Geometry: final body of the model. Coordinates: model frame, mm. A direction names the side the tool comes from. Coordinates: 2 decimals unless noted, no trailing zeros. Write each loop counter-clockwise with the first axis right and the second up, starting at its lowest first coordinate (ties: lowest second). Pieces come first, ordered by that corner, then holes. Notation, with made-up numbers: M 60.5,-12.75 L 108.5,-12.75 A30 ccw 108.5,23.25 Z; hole C 88.25,85.5 d5. An arc over 180 degrees is marked long. Write item = value, one per line. Start each with the question number.
Item 1: Reachability of faces 5 (the flat face through (96.71, 1, 3)), 6 (the flat face through (99, -30.344, 3)), 7 (the flat face through (85, 48.156, 3)) from +Z, -Z, +X, -X, +Y, -Y: full face, straight path, thin tool, end or side. Return the list, or none.
Item 2: First-contact query: pin 1 Ø3 at (x, z) = (85.5, 3.5) entering from -Y; pin 2 Ø1 at (x, z) = (-42.5, 4.5) entering from +Y; pin 3 Ø1.6 at (x, z) = (100, 4) entering from +Y; pin 4 Ø8 at (x, y) = (32.5, 30.5) entering from -Z. Flat tips, straight axial feed; report the tip coordinate or a pass-through.
Item 3: Pull-direction query (X, two-part tool) for faces 1 (the flat face through (-57.29, -20, 3)), 2 (the flat face through (39.21, 25, 3)), 3 (the flat face through (-60, 11.656, 3)), 4 (the flat face through (-31.79, -49, 3)); classes: +X half, -X half, draft (parallel to the pull), parting line (faces both ways), or undercut.
Item 4: Section A-A on y = 26. Output: boundary loops of the cut face in (x, z).
Item 5: Ray query, L1, parallel to Y at x = 43.5, z = 3.95; L2, parallel to X at y = 28, z = 4.05; L3, parallel to Y at x = 53, z = 3.3. Return the intervals inside material, ascending. Write a range as [from, to].
Item 6: Section C-C on z = 1.1. Give the number of separate pieces and of enclosed holes in the cut face, plus the area to 3 significant figures.
Item 7: Section D-D on y = 38.5. Output: boundary loops of the cut face in (x, z), plus the area to 3 significant figures.
Item 8: Section B-B on x = 85. Output: boundary loops of the cut face in (y, z).
from build123d import *

# Parameters (mm, degrees)
CROQUIS2_W              = 21
CROQUIS2_H              = 5.5
CROQUIS2_W_2            = 15.5
SALIENTE_EXTRUIR1_DEPTH = 5.5
CROQUIS3_W              = 21
CROQUIS3_H              = 5.5
CROQUIS3_W_2            = 7.5
SALIENTE_EXTRUIR2_DEPTH = 2.5
CROQUIS4_W              = 5.5
CROQUIS4_H              = 18.5
CROQUIS4_H_2            = 21
SALIENTE_EXTRUIR3_DEPTH = 2.5
CROQUIS5_W              = 10
CROQUIS5_H              = 5.5
CROQUIS5_W_2            = 21
SALIENTE_EXTRUIR4_DEPTH = 2.5
CROQUIS6_W              = 5.5
CROQUIS6_H              = 21
SALIENTE_EXTRUIR5_DEPTH = 2.5


with BuildPart() as part:
    # Croquis2 → Saliente-Extruir1 (new body)
    with BuildSketch(Plane.XY):
        Polygon((-60.290430527, -48.844252157), (-52.790430527, -48.844252157), (-52.790430527, -45.844252157), (-31.790430527, -45.844252157), (-31.790430527, -48.844252157), (-10.790430527, -48.844252157), (-10.790430527, -45.844252157), (10.209569473, -45.844252157), (10.209569473, -48.844252157), (31.209569473, -48.844252157), (31.209569473, -45.844252157), (52.209569473, -45.844252157), (52.209569473, -48.844252157), (73.209569473, -48.844252157), (73.209569473, -45.844252157), (94.209569473, -45.844252157), (96.709569473, -45.844252157), (96.709569473, -30.344252157), (99.709569473, -30.344252157), (99.709569473, -9.344252157), (96.709569473, -9.344252157), (96.709569473, 11.655747843), (99.709569473, 11.655747843), (99.709569473, 32.655747843), (96.709569473, 32.655747843), (96.709569473, 48.155747843), (73.209569473, 48.155747843), (73.209569473, 51.155747843), (52.209569473, 51.155747843), (52.209569473, 48.155747843), (31.209569473, 48.155747843), (31.209569473, 51.155747843), (10.209569473, 51.155747843), (10.209569473, 48.155747843), (-10.790430527, 48.155747843), (-10.790430527, 51.155747843), (-31.790430527, 51.155747843), (-31.790430527, 48.155747843), (-52.790430527, 48.155747843), (-52.790430527, 51.155747843), (-60.290430527, 51.155747843), (-60.290430527, 32.655747843), (-57.290430527, 32.655747843), (-57.290430527, 11.655747843), (-60.290430527, 11.655747843), (-60.290430527, -9.344252157), (-57.290430527, -9.344252157), (-57.290430527, -30.344252157), (-60.290430527, -30.344252157), align=None)
        with Locations((49.709569473, 25.315747843)):
            Rectangle(CROQUIS2_W, CROQUIS2_H, mode=Mode.SUBTRACT)
        with Locations((88.959569473, 25.315747843)):
            Rectangle(CROQUIS2_W_2, CROQUIS2_H, mode=Mode.SUBTRACT)
    extrude(amount=SALIENTE_EXTRUIR1_DEPTH)

    # Croquis3 → Saliente-Extruir2 (add)
    with BuildSketch(Plane(origin=(0, 51.155747843, 0), x_dir=(1, 0, 0), z_dir=(0, 1, 0))):
        with Locations((62.709569473, -2.75)):
            Rectangle(CROQUIS3_W, CROQUIS3_H)
        with Locations((20.709569473, -2.75)):
            Rectangle(CROQUIS3_W, CROQUIS3_H)
        with Locations((-21.290430527, -2.75)):
            Rectangle(CROQUIS3_W, CROQUIS3_H)
        with Locations((-56.540430527, -2.75)):
            Rectangle(CROQUIS3_W_2, CROQUIS3_H)
    extrude(amount=SALIENTE_EXTRUIR2_DEPTH)

    # Croquis4 → Saliente-Extruir3 (add)
    with BuildSketch(Plane.ZY.offset(60.290430527)):
        with Locations((2.75, -39.594252157)):
            Rectangle(CROQUIS4_W, CROQUIS4_H)
        with Locations((2.75, 1.155747843)):
            Rectangle(CROQUIS4_W, CROQUIS4_H_2)
        with Locations((2.75, 43.155747843)):
            Rectangle(CROQUIS4_W, CROQUIS4_H_2)
    extrude(amount=SALIENTE_EXTRUIR3_DEPTH)

    # Croquis5 → Saliente-Extruir4 (add)
    with BuildSketch(Plane.XZ.offset(48.844252157)):
        with Locations((-57.790430527, 2.75)):
            Rectangle(CROQUIS5_W, CROQUIS5_H)
        with Locations((-21.290430527, 2.75)):
            Rectangle(CROQUIS5_W_2, CROQUIS5_H)
        with Locations((20.709569473, 2.75)):
            Rectangle(CROQUIS5_W_2, CROQUIS5_H)
        with Locations((62.709569473, 2.75)):
            Rectangle(CROQUIS5_W_2, CROQUIS5_H)
    extrude(amount=SALIENTE_EXTRUIR4_DEPTH)

    # Croquis6 → Saliente-Extruir5 (add)
    with BuildSketch(Plane(origin=(99.709569473, 0, 0), x_dir=(0, 0, -1), z_dir=(1, 0, 0))):
        with Locations((-2.75, 22.155747843)):
            Rectangle(CROQUIS6_W, CROQUIS6_H)
        with Locations((-2.75, -19.844252157)):
            Rectangle(CROQUIS6_W, CROQUIS6_H)
    extrude(amount=SALIENTE_EXTRUIR5_DEPTH)


solid = part.part
Responses:
q1.face_5 = +Z, -Z, +X
q1.face_6 = +Z, -Z, +X, -Y
q1.face_7 = +Z, -Z, +X, +Y
q2.pin_1 = -45.84
q2.pin_2 = 48.16
q2.pin_3 = 32.66
q2.pin_4 = 0
q3.face_1 = -X half
q3.face_2 = undercut
q3.face_3 = draft
q3.face_4 = undercut
q4.outline = M -57.29,0 L 39.21,0 L 39.21,5.5 L -57.29,5.5 Z; M 60.21,0 L 81.21,0 L 81.21,5.5 L 60.21,5.5 Z; M 96.71,0 L 102.21,0 L 102.21,5.5 L 96.71,5.5 Z
q5.L1 = [-45.84, 22.57], [28.07, 48.16]
q5.L2 = [-57.29, 39.21], [60.21, 81.21], [96.71, 102.21]
q5.L3 = [-51.34, 22.57], [28.07, 53.66]
q6.separate_pieces = 1
q6.enclosed_holes = 2
q6.area = 15,600 mm²
q7.outline = M -62.79,0 L 96.71,0 L 96.71,5.5 L -62.79,5.5 Z
q7.area = 877 mm²
q8.outline = M -45.84,0 L 22.57,0 L 22.57,5.5 L -45.84,5.5 Z; M 28.07,0 L 48.16,0 L 48.16,5.5 L 28.07,5.5 Z
